```python
from build123d import *

# Parameters (mm, degrees)
SKETCH1_R               = 23.8
BOSS_EXTRUDE1_DEPTH     = 2.3
SKETCH2_R               = 23.8
SKETCH2_R_2             = 20.2
BOSS_EXTRUDE2_DEPTH     = 10
SKETCH3_R               = 3
BOSS_EXTRUDE3_DEPTH     = 17
CHAMFER1_SIZE           = 6
CHAMFER1_SIZE2          = 1.057961884
SKETCH4_R               = 1.25
CUT_EXTRUDE1_DEPTH      = 15
CUT_EXTRUDE3_START      = -9.2
SKETCH6_R               = 22.5
SKETCH6_R_2             = 20.2
CUT_EXTRUDE3_DEPTH      = 9.2
SKETCH7_R               = 1.5
CUT_EXTRUDE4_DEPTH      = 5
REDONDEO1_R             = 1.2
SALIENTE_EXTRUIR1_START = 1.6
CROQUIS1_R              = 9.339254136
CROQUIS1_R_2            = 1.25
SALIENTE_EXTRUIR1_DEPTH = 1.6
CROQUIS2_R              = 2
SALIENTE_EXTRUIR2_DEPTH = 3
CROQUIS4_R              = 4.654338303
CORTAR_EXTRUIR1_DEPTH   = 2.35


with BuildPart() as part:
    # Sketch1 → Boss-Extrude1 (new body)
    with BuildSketch(Plane.XY):
        Circle(SKETCH1_R)
    extrude(amount=BOSS_EXTRUDE1_DEPTH)

    # Sketch2 → Boss-Extrude2 (add)
    with BuildSketch(Plane.XY.offset(2.3)):
        Circle(SKETCH2_R)
        Circle(SKETCH2_R_2, mode=Mode.SUBTRACT)
    extrude(amount=BOSS_EXTRUDE2_DEPTH)

    # Sketch3 → Boss-Extrude3 (add)
    with BuildSketch(Plane.XY.offset(2.3)):
        Circle(SKETCH3_R)
    extrude(amount=BOSS_EXTRUDE3_DEPTH)

    # Chamfer1
    chamfer1_edges = [part.edges().sort_by_distance(p)[0] for p in [
        (-23.8, 0, 0),
    ]]
    chamfer1_side = [part.faces().sort_by_distance(p)[0] for p in [
        (0, 0, 0),
    ]]
    chamfer(chamfer1_edges, length=CHAMFER1_SIZE, length2=CHAMFER1_SIZE2, reference=chamfer1_side[0])

    # Sketch4 → Cut-Extrude1 (cut)
    with BuildSketch(Plane(origin=(0, 0, 0), x_dir=(-1, 0, 0), z_dir=(0, 0, -1))):
        with Locations((6, 0)):
            Circle(SKETCH4_R)
        with Locations((0, -6)):
            Circle(SKETCH4_R)
        with Locations((-6, 0)):
            Circle(SKETCH4_R)
        with Locations((0, 6)):
            Circle(SKETCH4_R)
    extrude(amount=-CUT_EXTRUDE1_DEPTH, mode=Mode.SUBTRACT)

    # Sketch6 → Cut-Extrude3 (cut)
    with BuildSketch(Plane.XY.offset(12.3).offset(CUT_EXTRUDE3_START)):
        Circle(SKETCH6_R)
        Circle(SKETCH6_R_2, mode=Mode.SUBTRACT)
    extrude(amount=CUT_EXTRUDE3_DEPTH, mode=Mode.SUBTRACT)

    # Sketch7 → Cut-Extrude4 (cut)
    with BuildSketch(Plane.XY.offset(19.3)):
        Circle(SKETCH7_R)
    extrude(amount=-CUT_EXTRUDE4_DEPTH, mode=Mode.SUBTRACT)

    # Redondeo1
    redondeo1_edges = [part.edges().sort_by_distance(p)[0] for p in [
        (-3, 0, 2.3),
    ]]
    fillet(redondeo1_edges, radius=REDONDEO1_R)

    # Croquis1 → Saliente-Extruir1 (add)
    with BuildSketch(Plane(origin=(0, 0, 0), x_dir=(-1, 0, 0), z_dir=(0, 0, -1)).offset(SALIENTE_EXTRUIR1_START)):
        Circle(CROQUIS1_R)
        with Locations((0, 6)):
            Circle(CROQUIS1_R_2, mode=Mode.SUBTRACT)
        with Locations((6, 0)):
            Circle(CROQUIS1_R_2, mode=Mode.SUBTRACT)
        with Locations((0, -6)):
            Circle(CROQUIS1_R_2, mode=Mode.SUBTRACT)
        with Locations((-6, 0)):
            Circle(CROQUIS1_R_2, mode=Mode.SUBTRACT)
    extrude(amount=-SALIENTE_EXTRUIR1_DEPTH)

    # Croquis2 → Saliente-Extruir2 (add)
    with BuildSketch(Plane(origin=(0, 0, -1.6), x_dir=(-1, 0, 0), z_dir=(0, 0, -1))):
        Circle(CROQUIS2_R)
    extrude(amount=SALIENTE_EXTRUIR2_DEPTH)

    # Croquis4 → Cortar-Extruir1 (cut)
    with BuildSketch(Plane(origin=(0, 0, -4.6), x_dir=(-1, 0, 0), z_dir=(0, 0, -1))):
        Circle(CROQUIS4_R)
    extrude(amount=-CORTAR_EXTRUIR1_DEPTH, mode=Mode.SUBTRACT)


solid = part.part
```
Could you check a few things on this model? Use its own coordinates, in mm. A direction names the side the tool comes from. Give positions to 0.01 mm unless a question says otherwise; leave off trailing zeros. Order: outer loops, then holes, each group sorted by start corner. A loop starts at its lowest first (then second) coordinate and runs counter-clockwise, first axis right, second up.
Q1. Suppose I cut it at B-B, the plane x = 0. Count the separate pieces of the cut face and the enclosed holes in it, and give its area (3 significant figures).
Q2. I'm going to push flat-ended pins straight in: P1, Ø3, axis at x = 6, y = 0, coming from the -Z side; P2, Ø2, axis at x = -15.5, z = 10.5, coming from the -Y side; P3, Ø12, axis at x = 7.5, z = 0.5, coming from the -Y side. Where does each tip first touch, or does it pass through?
Q3. For faces 4 (the cylindrical face through (0, -2, -2)), 5 (the flat face through (4, -4, 2.3)), 6 (the cylindrical face through (0.27, 4.78, 0.32)), which set-ups out of +Z, -Z, +X, -X, +Y, -Y let a thin tool reach every point of the face, with its end or its side?
Q4. If I drill on line 1 along Z through (x, y) = (-6, -11); line 2 along Y through (x, z) = (0, 13); line 3 along X through (y, z) = (-16.5, 3.5), over which ranges is the centre line in solid material (lowest first)?
Q5. Suppose I cut it at A-A, the plane z = 10.25. Write out the boundary of the cut face in (x, y), and give its area (3 significant figures).
Q6. We'd pull the mould along Y, two halves only. Please class faces 1 (the conical face through (-3.94, -17.743, 0.066)), 2 (the flat face through (-14, -18, 12.3)), 3 (the cylindrical face through (-3, 0, 11)): +Y half, -Y half, draft (parallel to the pull), parting line (faces both ways), or undercut.
Solution:
1. separate pieces: 3
1. enclosed holes: 0
1. area: 233 mm2
2. P1: stops at z = -1.6
2. P2: stops at y = -18.87
2. P3: stops at y = -23.75
3. face 4: -Z
3. face 5: +Z
3. face 6: +Z, -Z
4. line 1: z = 0 to 2.3
4. line 2: y = -3 to 3
4. line 3: x = -17.15 to -15.3, 15.3 to 17.15
5. outline: circle Ø47.6 at (0, 0); circle Ø6 at (0, 0); hole circle Ø45 at (0, 0)
5. area: 217 mm2
6. face 1: parting line
6. face 2: draft
6. face 3: undercut
